Read the model definition and answer for the solid it produces. Units are mm, in the model's axes. Face numbers are marked on the shaded views. A direction names the side the tool comes from. Coordinates: 2 decimals unless noted, no trailing zeros. Loops run counter-clockwise (first coordinate to the right, second up) from the corner with the lowest first, then second, coordinate; pieces in that order, holes last. Notation, with made-up numbers: (64.5, 2.25) -> (119.5, 2.25) arc R16 ccw to (119.5, 27.25) -> close; hole circle Ø1 at (-23.5, -5). An arc over 180 degrees is marked (long way). Answer as a JSON object with one key per item and string values. Group by question number.
1) Section B-B, the plane z = -0.75 is taken. Give the vertices of the cut face in (x, y), plus the area to 3 significant figures.
2) Section A-A, the plane x = 4.5 is taken. Give the vertices of the cut face in (y, z).
3) Section C-C, the plane z = 4.75 is taken. Give the vertices of the cut face in (x, y), plus the area to 3 significant figures.
4) Section D-D, the plane y = 25 is taken. Give the vertices of the cut face in (x, z).
5) Consider probe 1 along Z at (x, y) = (4.5, 3.85); probe 2 along X at (y, z) = (10, 4.75); probe 3 along Y at (x, z) = (32, 4). Determine where each line is inside the solid, lowest interval first. Write a range as [from, to].
6) Determine the mould class of the marked faces 5, 6 and 7 for opening direction Y: released by +Y, released by -Y, zero draft, split by the parting line, or undercut.
7) Which of the six approach directions +Z, -Z, +X, -X, +Y, -Y give full straight-line access (tool end or side, diameter ignored) to the marked faces 1, 2, 3 and 4?
8) Flat-ended cylindrical pins translate along their axes: P1, Ø2.5, axis at x = 50.5, z = 0, coming from the +Y side; P2, Ø3, axis at y = 32.5, z = -3, coming from the +X side; P3, Ø5.5, axis at x = 19, y = 30, coming from the +Z side; P4, Ø3, axis at y = 15, z = -3, coming from the +X side. Find the tip coordinate at first contact, or state that the pin passes through.
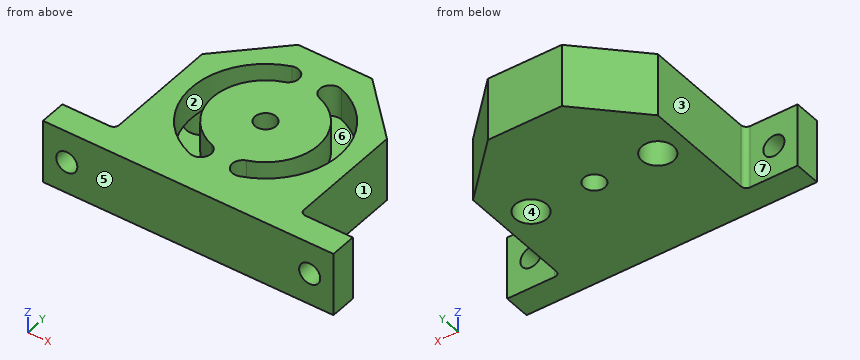
from build123d import *

# Parameters (mm, degrees)
BOSS_EXTRUDE1_DEPTH = 6
SKETCH2_R           = 2
CUT_EXTRUDE1_DEPTH  = 68.919069487
CUT_EXTRUDE2_DEPTH  = 6
SKETCH4_R           = 3
CUT_EXTRUDE3_DEPTH  = 6
SKETCH5_R           = 2
CUT_EXTRUDE4_DEPTH  = 65.420493634
FILLET1_R           = 1


with BuildPart() as part:
    # Sketch1 → Boss-Extrude1 (new, symmetric)
    with BuildSketch(Plane.XY):
        Polygon((0, 0), (55, 0), (55, 5), (45, 5), (45, 27.5), (34.5, 38), (20.5, 38), (10, 27.5), (10, 5), (0, 5), align=None)
    extrude(amount=BOSS_EXTRUDE1_DEPTH, both=True)

    # Sketch2 → Cut-Extrude1 (cut, through all)
    with BuildSketch(Plane.XY.offset(6)):
        with Locations((27.5, 20)):
            Circle(SKETCH2_R)
    extrude(amount=-CUT_EXTRUDE1_DEPTH, mode=Mode.SUBTRACT)

    # Sketch3 → Cut-Extrude2 (cut)
    with BuildSketch(Plane.XY.offset(6)):
        with BuildLine():
            ThreePointArc((24.166666667, 29.428090416), (17.5, 20), (24.166666667, 10.571909584))
            ThreePointArc((24.166666667, 10.571909584), (25.385618083, 8.019624834), (22.833333333, 6.800673418))
            ThreePointArc((22.833333333, 6.800673418), (13.5, 20), (22.833333333, 33.199326582))
            ThreePointArc((22.833333333, 33.199326582), (25.385618083, 31.980375166), (24.166666667, 29.428090416))
        make_face()
        with BuildLine():
            ThreePointArc((32.166666667, 6.800673418), (29.614381917, 8.019624834), (30.833333333, 10.571909584))
            ThreePointArc((30.833333333, 10.571909584), (37.5, 20), (30.833333333, 29.428090416))
            ThreePointArc((30.833333333, 29.428090416), (29.614381917, 31.980375166), (32.166666667, 33.199326582))
            ThreePointArc((32.166666667, 33.199326582), (41.5, 20), (32.166666667, 6.800673418))
        make_face()
    extrude(amount=-CUT_EXTRUDE2_DEPTH, mode=Mode.SUBTRACT)

    # Sketch4 → Cut-Extrude3 (cut)
    with BuildSketch(Plane(origin=(0, 0, -6), x_dir=(-1, 0, 0), z_dir=(0, 0, -1))):
        with Locations((-39.5, 20)):
            Circle(SKETCH4_R)
        with Locations((-15.5, 20)):
            Circle(SKETCH4_R)
    extrude(amount=-CUT_EXTRUDE3_DEPTH, mode=Mode.SUBTRACT)

    # Sketch5 → Cut-Extrude4 (cut, through all)
    with BuildSketch(Plane(origin=(0, 5, 0), x_dir=(1, 0, 0), z_dir=(0, 1, 0))):
        with Locations(Location((4.5, 0, 0), (0, 0, 180))):
            Circle(SKETCH5_R)
        with Locations(Location((50.5, 0, 0), (0, 0, 180))):
            Circle(SKETCH5_R)
    extrude(amount=-CUT_EXTRUDE4_DEPTH, mode=Mode.SUBTRACT)

    # Fillet1
    fillet1_edges = [part.edges().sort_by_distance(p)[0] for p in [
        (10, 5, 0),
        (45, 5, 0),
    ]]
    fillet(fillet1_edges, radius=FILLET1_R)


solid = part.part
Determined:
{
 "1": {"outline": "(0, 0) -> (2.65, 0) -> (2.65, 5) -> (0, 5) -> close; (6.35, 0) -> (48.65, 0) -> (48.65, 5) -> (46, 5) arc R1 cw to (45, 6) -> (45, 27.5) -> (34.5, 38) -> (20.5, 38) -> (10, 27.5) -> (10, 6) arc R1 cw to (9, 5) -> (6.35, 5) -> close; (52.35, 0) -> (55, 0) -> (55, 5) -> (52.35, 5) -> close; hole circle Ø6 at (15.5, 20); hole circle Ø4 at (27.5, 20); hole circle Ø6 at (39.5, 20)", "area": "1,210 mm²"},
 "2": {"outline": "(0, -6) -> (5, -6) -> (5, -2) -> (0, -2) -> close; (0, 2) -> (5, 2) -> (5, 6) -> (0, 6) -> close"},
 "3": {"outline": "(0, 0) -> (55, 0) -> (55, 5) -> (46, 5) arc R1 cw to (45, 6) -> (45, 27.5) -> (34.5, 38) -> (20.5, 38) -> (10, 27.5) -> (10, 6) arc R1 cw to (9, 5) -> (0, 5) -> close; hole (22.83, 6.8) arc R2 ccw to (24.17, 10.57) arc R10 cw to (24.17, 29.43) arc R2 ccw to (22.83, 33.2) arc R14 ccw to start; hole circle Ø4 at (27.5, 20); hole (30.83, 10.57) arc R2 ccw to (32.17, 6.8) arc R14 ccw to (32.17, 33.2) arc R2 ccw to (30.83, 29.43) arc R10 cw to start", "area": "1,050 mm²"},
 "4": {"outline": "(10, -6) -> (45, -6) -> (45, 6) -> (40.58, 6) -> (40.58, 0) -> (36.16, 0) -> (36.16, 6) -> (18.84, 6) -> (18.84, 0) -> (14.42, 0) -> (14.42, 6) -> (10, 6) -> close"},
 "5": {"probe 1": "[-6, -2], [2, 6]", "probe 2": "[10, 17.7], [25.01, 29.99], [37.3, 45]", "probe 3": "[0, 6.75], [11.07, 28.93], [33.25, 38]"},
 "6": {"face 5": "released by -Y", "face 6": "undercut", "face 7": "released by +Y"},
 "7": {"face 1": "+Z, -Z, +X, +Y", "face 2": "+Z", "face 3": "+Z, -Z, -X, +Y", "face 4": "-Z"},
 "8": {"P1": "through", "P2": "x = 41.5", "P3": "z = 6", "P4": "x = 45"}
}
